Build history of the part. All positions in model axes, mm. Face numbers are marked on the shaded views. A direction names the side the tool comes from. Round coordinates to 2 decimals unless told otherwise and drop trailing zeros. Write each loop counter-clockwise with the first axis right and the second up, starting at its lowest first coordinate (ties: lowest second). Pieces come first, ordered by that corner, then holes. Notation, with made-up numbers: (-12.75, 86) - (5.25, 86) arc R31 cw to (5.25, 112) - close; hole circle Ø10 at (22, 77). An arc over 180 degrees is marked (long way). Write each question's results on one line, items separated by ' | '.
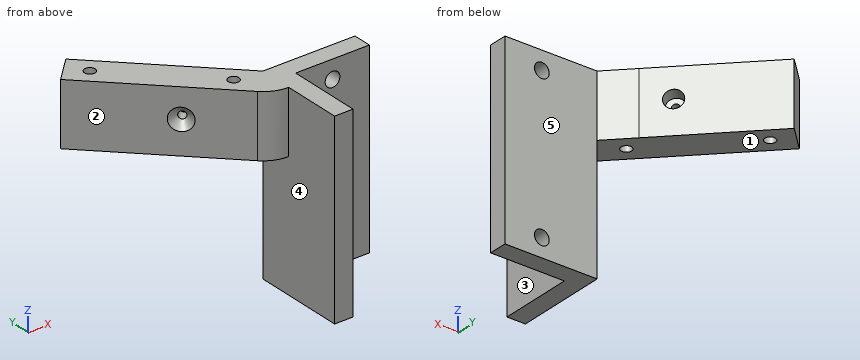
from build123d import *

# Parameters (mm, degrees)
F0_R     = 1.45
F1_DEPTH = 17
F2_DEPTH = 51
F3_R     = 1
F4_DEPTH = 43.4286695297
F3_R_2   = 2.4
F5_DEPTH = 4
F6_SIZE  = 2
F7_R     = 2
F8_DEPTH = 25.001


# Not quite as in the source:
# - a feature names something its author has since deleted; it is built from what else it names


with BuildPart() as f1:
    # F0 (on Top) → F1 (new body)
    with BuildSketch(Plane.XY):
        with BuildLine():
            ThreePointArc((-6.2514946472, 3.0411327703), (-8.8875336165, 9.4050938009), (-6.2514946472, 15.7690548316))
            Line((-6.2514946472, 15.7690548316), (-29.9395718169, 39.4571320014))
            Line((-29.9395718169, 39.4571320014), (-36.3035328476, 33.0931709707))
            Line((-36.3035328476, 33.0931709707), (-6.2514946472, 3.0411327703))
        make_face()
        with Locations((-29.0556883405, 32.2092874942)):
            Circle(F0_R, mode=Mode.SUBTRACT)
        with BuildLine():
            Line((-6.2514946472, 3.0411327703), (0.1124663835, 9.4050938009))
            Line((0.1124663835, 9.4050938009), (-6.2514946472, 15.7690548316))
            ThreePointArc((-6.2514946472, 15.7690548316), (-8.8875336165, 9.4050938009), (-6.2514946472, 3.0411327703))
        make_face()
        with Locations((-7.1353781237, 10.2889772774)):
            Circle(F0_R, mode=Mode.SUBTRACT)
        with BuildLine():
            Line((0.1124663835, 0.4050938009), (0.1124663835, 9.4050938009))
            Line((0.1124663835, 9.4050938009), (-6.2514946472, 3.0411327703))
            ThreePointArc((-6.2514946472, 3.0411327703), (-3.3316845078, 1.0901780083), (0.1124663835, 0.4050938009))
        make_face()
    extrude(amount=-F1_DEPTH)

    # F0 (on Top) → F2 (join)
    with BuildSketch(Plane.XY):
        with BuildLine():
            ThreePointArc((5.1124663835, 1.9217790274), (2.7249524636, 0.7926077208), (0.1124663835, 0.4050938009))
            Line((0.1124663835, 0.4050938009), (0.1124663835, -15.5949061991))
            Line((0.1124663835, -15.5949061991), (5.1124663835, -15.5949061991))
            Line((5.1124663835, -15.5949061991), (5.1124663835, 1.9217790274))
        make_face()
        with BuildLine():
            Line((9.1124663835, 9.4050938009), (0.1124663835, 9.4050938009))
            Line((0.1124663835, 9.4050938009), (0.1124663835, 0.4050938009))
            ThreePointArc((0.1124663835, 0.4050938009), (2.7249524636, 0.7926077208), (5.1124663835, 1.9217790274))
            Line((5.1124663835, 1.9217790274), (5.1124663835, 4.4050938009))
            Line((5.1124663835, 4.4050938009), (7.595781157, 4.4050938009))
            ThreePointArc((7.595781157, 4.4050938009), (8.7249524636, 6.7926077208), (9.1124663835, 9.4050938009))
        make_face()
        with BuildLine():
            Line((25.1124663835, 9.4050938009), (9.1124663835, 9.4050938009))
            ThreePointArc((9.1124663835, 9.4050938009), (8.7249524636, 6.7926077208), (7.595781157, 4.4050938009))
            Line((7.595781157, 4.4050938009), (25.1124663835, 4.4050938009))
            Line((25.1124663835, 4.4050938009), (25.1124663835, 9.4050938009))
        make_face()
    extrude(amount=-F2_DEPTH)

    # F3 (on face) → F4 (cut, through all)
    with BuildSketch(Plane(origin=(4.7587800922, 4.7587800922, 0), x_dir=(-0.7071067812, 0.7071067812, 0), z_dir=(0.7071067812, 0.7071067812, 0))):
        with Locations((23.0708798619, -8)):
            Circle(F3_R)
    extrude(amount=-F4_DEPTH, mode=Mode.SUBTRACT)

    # F3 (on face) → F5 (cut)
    with BuildSketch(Plane(origin=(4.7587800922, 4.7587800922, 0), x_dir=(-0.7071067812, 0.7071067812, 0), z_dir=(0.7071067812, 0.7071067812, 0))):
        with Locations((23.0708798619, -8)):
            Circle(F3_R_2)
        with Locations((23.0708798619, -8)):
            Circle(F3_R, mode=Mode.SUBTRACT)
    extrude(amount=-F5_DEPTH, mode=Mode.SUBTRACT)

    # F6
    f6_edges = [f1.edges().sort_by_distance(p)[0] for p in [
        (-17.21165, 14.001288, -8),
    ]]
    chamfer(f6_edges, length=F6_SIZE)

    # F7 (on face) → F8 (cut, through all)
    with BuildSketch(Plane(origin=(0, 9.4050938009, 0), x_dir=(-1, 0, 0), z_dir=(0, 1, 0))):
        with Locations((-15.1124663835, -5)):
            Circle(F7_R)
        with Locations((-15.1124663835, -46)):
            Circle(F7_R)
    extrude(amount=-F8_DEPTH, mode=Mode.SUBTRACT)


solid = f1.part
(1) Slice it at A-A, the plane z = -46. Write the cut outline in (x, y), and give its area (3 significant figures).
Worked answers:
outline: (0.11, -15.59) - (5.11, -15.59) - (5.11, 4.41) - (13.11, 4.41) - (13.11, 9.41) - (0.11, 9.41) - close; (17.11, 4.41) - (25.11, 4.41) - (25.11, 9.41) - (17.11, 9.41) - close | area: 205 mm2
(2) Tool access for the marked faces 1, 2, 3, 4 and 5: list every direction of +Z, -Z, +X, -X, +Y, -Y with a clear straight run to the whole face (end or side of a thin tool).
Worked answers:
face 1: -Z, -X, +Y, -Y | face 2: +Z, -Z, -X, -Y | face 3: +Z, -Z, +X, -Y | face 4: -Z, -X, -Y | face 5: +Z, -Z, +X, +Y
(3) Slice it at D-D, the plane x = 10. Write the cut outline in (y, z), and give its area (3 significant figures).
Worked answers:
outline: (4.41, -51) - (9.41, -51) - (9.41, 0) - (4.41, 0) - close | area: 255 mm2
(4) Drill centre lines: probe 1 along Y at (x, z) = (4, -24.5); probe 2 along X at (y, z) = (-10.5, -11); probe 3 along Y at (x, z) = (16.5, -41.5). Where is each one in solid material? Low to high. Write a range as [from, to].
Worked answers:
probe 1: y = [-15.59, 9.41] | probe 2: x = [0.11, 5.11] | probe 3: y = [4.41, 9.41]
(5) Slice it at C-C, the plane y = -8.5. Write the cut outline in (x, z).
Worked answers:
outline: (0.11, -51) - (5.11, -51) - (5.11, 0) - (0.11, 0) - close
(6) Flat gauge pins, fed straight in: pin 1 Ø2.5 at (x, y) = (-29.06, 32.21) entering from +Z; pin 2 Ø7.5 at (y, z) = (-3, -37) entering from -X; pin 3 Ø7.5 at (x, z) = (16.5, -22) entering from +Y; pin 4 Ø2 at (x, y) = (9.5, 4.5) entering from +Z. Where does each tip first touch, or does it go through?
Worked answers:
pin 1: passes through | pin 2: stops at x = 0.11 | pin 3: stops at y = 9.41 | pin 4: stops at z = 0
(7) Slice it at B-B, the plane x = -29. Write the cut outline in (y, z), and give its area (3 significant figures).
Worked answers:
outline: (25.79, -17) - (30.76, -17) - (30.76, 0) - (25.79, 0) - close; (33.66, -17) - (38.52, -17) - (38.52, 0) - (33.66, 0) - close | area: 167 mm2
